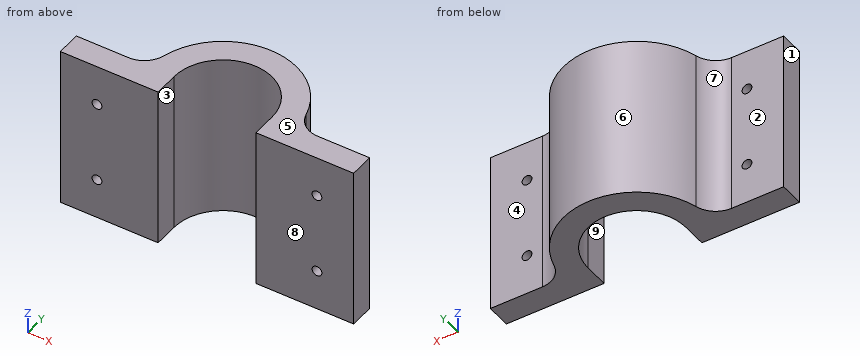
from build123d import *

# Parameters (mm, degrees)
F1_DEPTH = 20
F3_D     = 1.2
F4_R     = 3


with BuildPart() as f1:
    # F0 (on Top) → F1 (new body)
    with BuildSketch(Plane.XY):
        with BuildLine():
            ThreePointArc((-6, 0), (0, 6), (6, 0))
            Line((6, 0), (6, -3))
            Line((6, -3), (18, -3))
            Line((18, -3), (18, 0))
            Line((18, 0), (9, 0))
            ThreePointArc((9, 0), (0, 9), (-9, 0))
            Line((-9, 0), (-18, 0))
            Line((-18, 0), (-18, -3))
            Line((-18, -3), (-6, -3))
            Line((-6, -3), (-6, 0))
        make_face()
    extrude(amount=F1_DEPTH)

    # F3 (through all)
    with Locations(Plane(origin=(0, 0, 0), x_dir=(-1, 0, 0), z_dir=(0, 1, 0))):
        with Locations((-13.5, 15), (-13.5, 5), (13.5, 15), (13.5, 5)):
            Hole(F3_D / 2)

    # F4
    f4_edges = [f1.edges().sort_by_distance(p)[0] for p in [
        (9, 0, 10),
        (-9, 0, 10),
    ]]
    fillet(f4_edges, radius=F4_R)


solid = f1.part
Geometry check sheet. Reference: the model listing, model coordinates, mm. Face numbers are marked on the shaded views. A direction names the side the tool comes from. Give positions to 0.01 mm unless a question says otherwise; leave off trailing zeros. Write each loop counter-clockwise with the first axis right and the second up, starting at its lowest first coordinate (ties: lowest second). Pieces come first, ordered by that corner, then holes. Notation, with made-up numbers: M -35,64.5 L -10,64.5 A26 ccw -10,94.5 Z; hole C -35.75,11.5 d1. An arc over 180 degrees is marked long. One line per question, with ' | ' between items.
1. Mould release check, pull along X, two halves, no side actions. Record for the marked faces 6, 7, 8 and 9: released by +X, released by -X, zero draft, split by the parting line, or undercut.
Ans:
face 6: split by the parting line | face 7: released by -X | face 8: zero draft | face 9: undercut
2. Cross-section at C-C (z = 15). Enter the section's corners in (x, y), plus the area to 3 significant figures.
Ans:
outline: M -18,-3 L -14.1,-3 L -14.1,0 L -18,0 Z; M -12.9,-3 L -6,-3 L -6,0 A6 cw 6,0 L 6,-3 L 12.9,-3 L 12.9,0 L 11.62,0 A3 cw 8.71,2.25 A9 ccw -8.71,2.25 A3 cw -11.62,0 L -12.9,0 Z; M 14.1,-3 L 18,-3 L 18,0 L 14.1,0 Z | area: 138 mm2
3. Cross-section at A-A (x = -13.5). Enter the section's corners in (y, z).
Ans:
outline: M -3,0 L 0,0 L 0,4.4 L -3,4.4 Z; M -3,5.6 L 0,5.6 L 0,14.4 L -3,14.4 Z; M -3,15.6 L 0,15.6 L 0,20 L -3,20 Z
4. Gauge pin test, flat ends, axial feed: pin 1 (5 mm diameter, centred on x = 10.5, y = 6, fed in from +Z); pin 2 (2 mm diameter, centred on y = 8, z = 4.5, fed in from -X); pin 3 (3 mm diameter, centred on y = 6.5, z = 7, fed in from +X); pin 4 (7 mm diameter, centred on x = 13.5, z = 10, fed in from +Y). Record the tip position at first contact, or that the pin passes through.
Ans:
pin 1: through | pin 2: x = -5.66 | pin 3: x = 7.48 | pin 4: y = 0.47
5. Scan lines: line 1 along Z through (x, y) = (13.5, -1.5); line 2 along X through (y, z) = (-1.5, 12.5); line 3 along Y through (x, z) = (-14, 1.75). Record each from-to range of solid material in increasing order. Write a range as from..to.
Ans:
line 1: 0..4.4, 5.6..14.4, 15.6..20 | line 2: -18..-6, 6..18 | line 3: -3..0
6. Cross-section at D-D (z = 9.75). Enter the section's corners in (x, y), plus the area to 3 significant figures.
Ans:
outline: M -18,-3 L -6,-3 L -6,0 A6 cw 6,0 L 6,-3 L 18,-3 L 18,0 L 11.62,0 A3 cw 8.71,2.25 A9 ccw -8.71,2.25 A3 cw -11.62,0 L -18,0 Z | area: 145 mm2
7. Set-up check for the marked faces 1, 2, 3, 4 and 5: record each of +Z, -Z, +X, -X, +Y, -Y from which the full face is reachable in a straight line by a thin tool's end or side.
Ans:
face 1: +Z, -Z, -X, +Y, -Y | face 2: +Z, -Z, -X, +Y | face 3: +Z, -Z, -Y | face 4: +Z, -Z, +X, +Y | face 5: +Z, +X, -X, +Y, -Y
8. Cross-section at B-B (y = -1.5). Enter the section's corners in (x, z).
Ans:
outline: M -18,0 L -6,0 L -6,20 L -18,20 Z; M 6,0 L 18,0 L 18,20 L 6,20 Z; hole C -13.5,5 d1.2; hole C -13.5,15 d1.2; hole C 13.5,5 d1.2; hole C 13.5,15 d1.2
